```python
from build123d import *

# Parameters (mm, degrees)
F0_R     = 12.5
F1_DEPTH = 25


with BuildPart() as f1:
    # F0 (on Top) → F1 (new body)
    with BuildSketch(Plane.XY):
        Circle(F0_R)
        with BuildLine():
            ThreePointArc((117.5, 0), (110, 7.5), (102.5, 0))
            ThreePointArc((102.5, 0), (110, -7.5), (117.5, 0))
        make_face()
        with BuildLine():
            ThreePointArc((-7.627142, 23.960834), (-8.490667, 23.55277), (-9.369148, 23.177987))
            ThreePointArc((-9.369148, 23.177987), (-19.916156, -15.111146), (19.798746, -15.264653))
            ThreePointArc((19.798746, -15.264653), (22.493335, -12.564186), (25.782002, -10.630792))
            ThreePointArc((25.782002, -10.630792), (60.546561, -3.019212), (95.672722, -8.734419))
            ThreePointArc((95.672722, -8.734419), (98.089359, -9.868623), (100.266669, -11.41325))
            ThreePointArc((100.266669, -11.41325), (122.489592, -8.307231), (116.763269, 13.388734))
            ThreePointArc((116.763269, 13.388734), (115.800812, 13.920051), (114.879855, 14.520434))
            ThreePointArc((114.879855, 14.520434), (54.926268, 36.109448), (-7.627142, 23.960834))
        make_face()
        Circle(F0_R, mode=Mode.SUBTRACT)
        with BuildLine():
            ThreePointArc((117.5, 0), (110, -7.5), (102.5, 0))
            ThreePointArc((102.5, 0), (110, 7.5), (117.5, 0))
        make_face(mode=Mode.SUBTRACT)
    extrude(amount=F1_DEPTH)


solid = f1.part
```
Here's how the part is built. I have some questions about the finished solid (model axes, mm). A direction names the side the tool comes from. Round coordinates to 2 decimals unless told otherwise and drop trailing zeros. Write each loop counter-clockwise with the first axis right and the second up, starting at its lowest first coordinate (ties: lowest second). Pieces come first, ordered by that corner, then holes. Notation, with made-up numbers: M 84.25,70.25 L 107.25,70.25 A13 cw 107.25,82.25 Z; hole C -21,60 d3. An arc over 180 degrees is marked long. Answer as CSV lines item,"result". Start each with the question number.
1. Suppose I cut it at B-B on y = 0. Write out the boundary of the cut face in (x, z), then the cut area to 3 significant figures.
2. Thinking about a two-plate mould opening in X: for faces 3 (the flat face through (49, 6, 0)), 4 (the cylindrical face through (98.06, -9.85, 12.32)), 5 (the cylindrical face through (55.826, 36.037, 12.325)), which applies, released by +X, released by -X, zero draft, split by the parting line, or undercut?
3. Suppose I cut it at D-D on x = 110. Write out the boundary of the cut face in (y, z).
4. Suppose I cut it at C-C on z = 19.25. Write out the boundary of the cut face in (x, y).
5. I need wall thicknesses on probe 1 along Y at (x, z) = (110, 7.75); probe 2 along Y at (x, z) = (0, 10); probe 3 along Y at (x, z) = (96, 2). Which ranges of each line are inside material? Lowest first, please.
6. Suppose I cut it at A-A on x = 0. Write out the boundary of the cut face in (y, z), then the cut area to 3 significant figures.
7. I'm going to push flat-ended pins straight in: pin 1 Ø10 at (x, z) = (36.5, 17.5) entering from +Y; pin 2 Ø2 at (y, z) = (28, 11.5) entering from +X; pin 3 Ø1.5 at (x, z) = (17, 10) entering from -Y. Where does each tip first touch, or does it pass through?
8. On a 3-axis mill with a long thin cutter (end or side, diameter ignored), from which of +Z, -Z, +X, -X, +Y, -Y can I reach the whole of each face in a straight line? I mean faces 1 (the cylindrical face through (102.846, 2.253, 12.325)), 2 (the cylindrical face through (22.45, -12.6, 12.32)). Say none if no direction works.
Check result:
1,outline,"M -25,0 L -12.5,0 L -12.5,25 L -25,25 Z; M 12.5,0 L 102.5,0 L 102.5,25 L 12.5,25 Z; M 117.5,0 L 125,0 L 125,25 L 117.5,25 Z"
1,area,"2,750 mm2"
2,face 3,"zero draft"
2,face 4,"undercut"
2,face 5,"split by the parting line"
3,outline,"M -15,0 L -7.5,0 L -7.5,25 L -15,25 Z; M 7.5,0 L 17.79,0 L 17.79,25 L 7.5,25 Z"
4,outline,"M -9.37,23.18 A25 ccw long 19.8,-15.26 A15 cw 25.78,-10.63 A95 cw 95.67,-8.73 A15 cw 100.27,-11.41 A15 ccw long 116.76,13.39 A15 cw 114.88,14.52 A120 ccw -7.63,23.96 A25 cw Z; hole C 0,0 d25; hole C 110,0 d15"
5,probe 1,"y = -15 to -7.5, 7.5 to 17.79"
5,probe 2,"y = -25 to -12.5, 12.5 to 27.42"
5,probe 3,"y = -8.86 to 25.42"
6,outline,"M -25,0 L -12.5,0 L -12.5,25 L -25,25 Z; M 12.5,0 L 27.42,0 L 27.42,25 L 12.5,25 Z"
6,area,"685 mm2"
7,pin 1,"stops at y = 36.39"
7,pin 2,"stops at x = 92.42"
7,pin 3,"stops at y = -19"
8,face 1,"+Z, -Z"
8,face 2,"+Z, -Z, -Y"
